Source: CAD feature listing. Evaluate the final solid. Frame: model axes, mm. Face numbers are marked on the shaded views. A direction names the side the tool comes from. Round coordinates to 2 decimals unless told otherwise and drop trailing zeros. Write each loop counter-clockwise with the first axis right and the second up, starting at its lowest first coordinate (ties: lowest second). Pieces come first, ordered by that corner, then holes.
from build123d import *

# Parameters (mm, degrees)
SKETCH1_W                 = 50
SKETCH1_H                 = 70
BOSS_EXTRUDE1_DEPTH       = 33.5
CUT_EXTRUDE2_DEPTH        = 1.5
SKETCH3_W                 = 29
SKETCH3_H                 = 3.3
CUT_EXTRUDE3_DEPTH        = 51
CUT_EXTRUDE4_DEPTH        = 51
F_6_0MM_DOWEL_HOLE2_D     = 6.3
F_6_0MM_DOWEL_HOLE2_DEPTH = 12.5
CUT_EXTRUDE6_DEPTH        = 1.5


with BuildPart() as part:
    # Sketch1 → Boss-Extrude1 (new body, symmetric)
    with BuildSketch(Plane.XY):
        with Locations((25, 35)):
            Rectangle(SKETCH1_W, SKETCH1_H)
    extrude(amount=BOSS_EXTRUDE1_DEPTH, both=True)

    # Sketch2 → Cut-Extrude2 (cut)
    with BuildSketch(Plane.XY.offset(33.5)):
        Polygon((19.101262674, 35), (25, 43.258232256), (5.898737326, 70), (0, 70), (0, 61.741767744), align=None)
        Polygon((50, 0), (50, 8.258232256), (30.898737326, 35), (25, 26.741767744), (44.101262674, 0), align=None)
        Polygon((25, 43.258232256), (30.898737326, 35), (50, 61.741767744), (50, 70), (44.101262674, 70), align=None)
        Polygon((5.898737326, 0), (25, 26.741767744), (19.101262674, 35), (0, 8.258232256), (0, 0), align=None)
        Polygon((25, 26.741767744), (30.898737326, 35), (25, 43.258232256), (19.101262674, 35), align=None)
    extrude(amount=-CUT_EXTRUDE2_DEPTH, mode=Mode.SUBTRACT)

    # Sketch3 → Cut-Extrude3 (cut, through all)
    with BuildSketch(Plane(origin=(50, 0, 0), x_dir=(0, 0, -1), z_dir=(1, 0, 0))):
        with Locations((19, 55.85)):
            Rectangle(SKETCH3_W, SKETCH3_H)
    extrude(amount=-CUT_EXTRUDE3_DEPTH, mode=Mode.SUBTRACT)

    # Sketch4 → Cut-Extrude4 (cut, through all)
    with BuildSketch(Plane(origin=(50, 0, 0), x_dir=(0, 0, -1), z_dir=(1, 0, 0))):
        with BuildLine():
            Line((33.5, 36.5), (9.954482672, 36.5))
            ThreePointArc((9.954482672, 36.5), (-25.5, 27), (9.954482672, 17.5))
            Line((9.954482672, 17.5), (33.5, 17.5))
            Line((33.5, 17.5), (33.5, 36.5))
        make_face()
    extrude(amount=-CUT_EXTRUDE4_DEPTH, mode=Mode.SUBTRACT)

    # Ø6.0mm Dowel Hole2
    with Locations(Plane(origin=(0, 70, 0), x_dir=(1, 0, 0), z_dir=(0, 1, 0))):
        with Locations((33.5, 25.2)):
            Hole(F_6_0MM_DOWEL_HOLE2_D / 2, depth=F_6_0MM_DOWEL_HOLE2_DEPTH)

    # Sketch15 → Cut-Extrude6 (cut)
    with BuildSketch(Plane(origin=(37.5, 0, 0), x_dir=(0, 0, -1), z_dir=(1, 0, 0))):
        with BuildLine():
            Line((9.954482672, 36.5), (11.099715907, 36.5))
            ThreePointArc((11.099715907, 36.5), (-26.5, 27), (11.099715907, 17.5))
            Line((11.099715907, 17.5), (9.954482672, 17.5))
            ThreePointArc((9.954482672, 17.5), (-25.5, 27), (9.954482672, 36.5))
        make_face()
    cut_extrude6 = extrude(amount=CUT_EXTRUDE6_DEPTH, mode=Mode.SUBTRACT)

    # Mirror2: Cut-Extrude6 across plane
    add(cut_extrude6.mirror(Plane(origin=(25, 0, 0), x_dir=(0, 0, 1), z_dir=(1, 0, 0))), mode=Mode.SUBTRACT)


solid = part.part
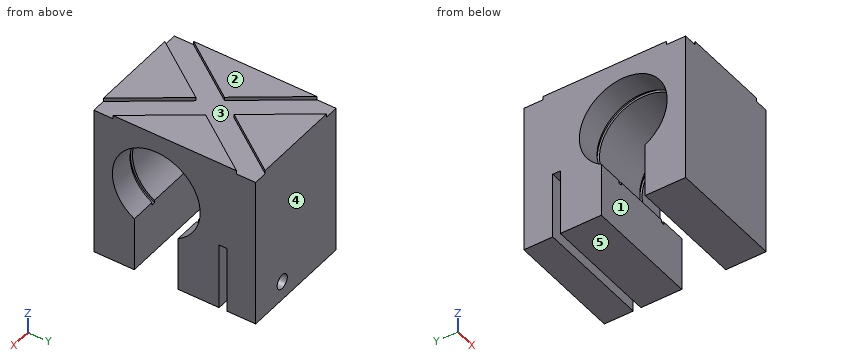
1) Section query D-D on y = 20. Return the cut outline in (x, z) (3 decimals).
Taken from the geometry:
outline: (0, 24.164) - (11, 24.164) - (11, 25.235) - (12.5, 25.235) - (12.5, 24.164) - (37.5, 24.164) - (37.5, 25.235) - (39, 25.235) - (39, 24.164) - (50, 24.164) - (50, 33.5) - (41.613, 33.5) - (41.613, 32) - (29.816, 32) - (29.816, 33.5) - (20.184, 33.5) - (20.184, 32) - (8.387, 32) - (8.387, 33.5) - (0, 33.5) - close
2) Section query C-C on x = 33.5. Return the cut outline in (y, z).
Taken from the geometry:
outline: (0, -33.5) - (17.5, -33.5) - (17.5, -9.95) arc R19 cw (long way) to (36.5, -9.95) - (36.5, -33.5) - (54.2, -33.5) - (54.2, -4.5) - (57.5, -4.5) - (57.5, -22.05) - (70, -22.05) - (70, 33.5) - (55.16, 33.5) - (55.16, 32) - (38.64, 32) - (38.64, 33.5) - (31.36, 33.5) - (31.36, 32) - (14.84, 32) - (14.84, 33.5) - (0, 33.5) - close; (57.5, -33.5) - (70, -33.5) - (70, -28.35) - (57.5, -28.35) - close
3) Pull-direction query (Y, two-part tool) for the marked faces 3, 4 and 5; classes: released by +Y, released by -Y, zero draft, split by the parting line, or undercut.
Taken from the geometry:
face 3: undercut
face 4: released by +Y
face 5: zero draft
4) Material intervals for line 1 (Y direction, x = 15, z = -20); line 2 (X direction, y = 65, z = -25); line 3 (Y direction, x = 11.85, z = 6.5), sorted ascending.
Taken from the geometry:
line 1: y = 0 to 17.5, 36.5 to 54.2, 57.5 to 70
line 2: x = 0 to 30.36, 36.64 to 50
line 3: y = 0 to 7, 47 to 70
5) Reachability of the marked faces 1 and 2 from +Z, -Z, +X, -X, +Y, -Y: full face, straight path, thin tool, end or side. Return the list, or none.
Taken from the geometry:
face 1: -Z, +X, -X
face 2: +Z, +X, -X, +Y, -Y
6) Section query A-A on z = 6.5. Return the cut outline in (x, y), then the cut area to 3 significant figures.
Taken from the geometry:
outline: (0, 0) - (50, 0) - (50, 8) - (39, 8) - (39, 7) - (37.5, 7) - (37.5, 8) - (12.5, 8) - (12.5, 7) - (11, 7) - (11, 8) - (0, 8) - close; (0, 46) - (11, 46) - (11, 47) - (12.5, 47) - (12.5, 46) - (37.5, 46) - (37.5, 47) - (39, 47) - (39, 46) - (50, 46) - (50, 70) - (0, 70) - close
area: 1,590 mm2
7) Contact query for flat-ended pins moving along their axis: P1, Ø2, axis at x = 22, y = 21, coming from the -Z side; P2, Ø2.5, axis at x = 30.5, y = 56, coming from the -Z side; P3, Ø1, axis at x = 7.5, y = 53.5, coming from the +Z side; P4, Ø11.5, axis at y = 23, z = -0.5, coming from the -X side. Output: stop coordinate, or through.
Taken from the geometry:
P1: stops at z = 24.16
P2: stops at z = -4.5
P3: stops at z = 32
P4: passes through
8) Section query B-B on z = -25.2. Return the cut outline in (x, y), then the cut area to 3 significant figures.
Taken from the geometry:
outline: (0, 0) - (50, 0) - (50, 17.5) - (0, 17.5) - close; (0, 36.5) - (50, 36.5) - (50, 54.2) - (0, 54.2) - close; (0, 57.5) - (30.35, 57.5) - (30.35, 70) - (0, 70) - close; (36.65, 57.5) - (50, 57.5) - (50, 70) - (36.65, 70) - close
area: 2,310 mm2
